Geometry check sheet. Reference: the model listing, model coordinates, mm. A direction names the side the tool comes from. Round coordinates to 2 decimals unless told otherwise and drop trailing zeros. Loops run counter-clockwise (first coordinate to the right, second up) from the corner with the lowest first, then second, coordinate; pieces in that order, holes last. Notation, with made-up numbers: (-6.5, -21) - (17.5, -21) arc R13 ccw to (17.5, 4) - close; hole circle Ø11 at (81.5, 87). An arc over 180 degrees is marked (long way). Write item = value, one per line.
Autodesk Inventor part; units mm, degrees
ref_plane "YZ Plane" through (0, 0, 0) normal (1, 0, 0) x (0, 1, 0)
ref_plane "XY Plane" through (0, 0, 0) normal (0, 0, 1) x (1, 0, 0)
sketch "Sketch1" plane through (0, 0, 0) normal (0, 0, 1) x (1, 0, 0)
  circle A0 centre (0, 0) radius 142.875
  circle A1 centre (0, 0) radius 149.225
  dimension "innerDiameter" = 285.75
  dimension "outerDiameter" = 298.45
extrude "Extrusion1" add sketch "Sketch1" along normal mid plane 19.05
sketch "Sketch2" plane through (0, 0, 0) normal (0, 0, 1) x (1, 0, 0)
  circle A0 centre (0, 0) radius 142.875 construction
  line L0 (0, 142.875) -> (0, 149.225) construction
  circle A1 centre (0, 0) radius 149.225 construction
  line L1 (0, 142.875) -> (44.45, 142.875)
  line L2 (44.45, 142.875) -> (44.45, 149.225)
  line L3 (44.45, 149.225) -> (19.05, 149.225)
  line L4 (0, 142.875) -> (-44.45, 142.875)
  line L5 (-44.45, 142.875) -> (-44.45, 149.225)
  line L6 (-44.45, 149.225) -> (19.05, 149.225)
  line L7 (371.6693, 35.081) -> (0, 0)
  dimension "halfBaseWidth" = 44.45
  dimension "baseThickness" = 6.35
  dimension "baseHeight" = 0
extrude "Extrusion2" add sketch "Sketch2" along normal mid plane 19.05
sketch "Sketch5" plane through (-44.45, 149.225, 9.525) normal (0, 1, 0) x (1, 0, 0)
  line L0 (0, 19.05) -> (0, 0)
  line L1 (88.9, 19.05) -> (88.9, 0)
  line L2 (0, 0) -> (88.9, 0)
  line L3 (88.9, 0) -> (88.9, 19.05)
  line L4 (88.9, 19.05) -> (0, 19.05)
  line L5 (0, 19.05) -> (0, 0)
  point P0 (44.45, 9.525)
  point P1 (0, 19.05)
extrude "Extrusion3" add sketch "Sketch5" along normal blind 63.5
sketch "Sketch7" plane through (0, 0, 9.525) normal (0, 0, 1) x (1, 0, 0)
  line L0 (-44.45, 142.875) -> (-44.45, 212.725)
  line L1 (-44.45, 212.725) -> (44.45, 212.725)
  line L2 (44.45, 142.875) -> (44.45, 212.725)
  line L3 (0, 212.725) -> (0, 149.1868) construction
  line L4 (-15.875, 197.104) -> (15.875, 197.104)
  line L5 (15.875, 197.104) -> (15.875, 206.375)
  line L6 (15.875, 206.375) -> (-15.875, 206.375)
  line L7 (-15.875, 206.375) -> (-15.875, 197.104)
  line L8 (-15.875, 197.104) -> (15.875, 206.375) construction
  line L9 (15.875, 197.104) -> (-15.875, 206.375) construction
  point P0 (0, 0)
  point P1 (-38.1, 144.2792)
  point P2 (38.1, 144.2792)
  point P3 (0, 201.7395)
  dimension "screwHoleWidth" = 31.75
  dimension "screwHoleHeight" = 9.271
  dimension "screwHoleSupportThickness" = 6.35
extrude "Extrusion4" cut sketch "Sketch7" against normal through all
sketch "Sketch6" plane through (-44.45, 212.725, 9.525) normal (0, 1, 0) x (1, 0, 0)
  point P0 (44.45, 9.525)
  point P1 (44.45, 9.525)
hole "Hole2" at (0, 212.725, 0) direction (0, -1, 0) diameter 6.7564 depth 6.35
ref_plane "Work Plane1" through (0, 0, 0) normal (-0.7071, 0.7071, 0) x (0, 0, 1)
ref_plane "Work Plane2" through (0, 0, 0) normal (0.7071, 0.7071, 0) x (0, 0, 1)
sketch "Sketch11" plane through (0, 0, 0) normal (0, 0, 1) x (1, 0, 0)
  arc A0 (-43.0678, 142.875) -> (43.0678, 142.875) centre (0, 0) ccw
  circle A1 centre (0, 0) radius 142.875
  line L0 (-214.9625, 214.9625) -> (217.3313, -217.3313)
  line L1 (-101.0279, 101.0279) -> (-96.5378, 105.518)
  line L2 (-101.0279, 101.0279) -> (-94.6779, 101.0279) construction
  line L3 (-96.5378, 105.518) -> (-114.4983, 123.4785)
  line L4 (-96.5378, 105.518) -> (-71.1378, 105.518) construction
  line L5 (-114.4983, 123.4785) -> (-118.9884, 118.9884)
  line L6 (-118.9884, 118.9884) -> (-101.0279, 101.0279)
  line L7 (-101.0279, 101.0279) -> (-105.518, 96.5378)
  line L8 (-105.518, 96.5378) -> (-123.4785, 114.4983)
  line L9 (-123.4785, 114.4983) -> (-118.9884, 118.9884)
  point P0 (38.1, 144.2792)
  point P1 (-38.1, 144.2792)
  point P2 (-109.9126, 100.9323)
  point P3 (-100.9323, 109.9126)
  dimension "d47" = 6.35
  dimension "d48" = 45
  dimension "d49" = 25.4
  dimension "d50" = 135
extrude "Extrusion7" add sketch "Sketch11" along normal mid plane 19.05 contours A0 L0 L5 L3 | A0 L8 L9 L0
sketch "Sketch12" plane through (-114.4983, 123.4785, -9.525) normal (0.7071, 0.7071, 0) x (-0.7071, 0.7071, 0)
  line L0 (0, 0) -> (0, 19.05)
  line L1 (-19.1852, 19.05) -> (0, 19.05)
  line L2 (-19.1852, 0) -> (-19.1852, 19.05)
  line L3 (0, 0) -> (-19.1852, 0)
  line L4 (-9.5926, 19.05) -> (-9.5926, 0) construction
  line L5 (0, 9.525) -> (-19.1852, 9.525) construction
  point P0 (-168.275, 9.525)
  point P1 (-9.5926, 9.525)
hole "Hole4" at (-107.7153, 116.6955, 0) direction (-0.7071, -0.7071, 0) diameter 5.1054 depth 12.7
pattern_circular "Circular Pattern1" count 4 over 360 about axis through (0, 0, -10) along (0, 0, 1) of "Extrusion7", "Hole4"
sketch "Sketch13" plane through (0, 0, 9.525) normal (0, 0, 1) x (1, 0, 0)
  line L0 (-15.875, 206.375) -> (15.875, 206.375)
  line L1 (-44.45, 212.725) -> (44.45, 212.725)
  line L2 (0, 208.915) -> (8.89, 208.915)
  line L3 (8.89, 208.915) -> (8.89, 206.375)
  line L4 (8.89, 206.375) -> (0, 206.375)
  line L5 (0, 208.915) -> (0, 206.375)
  line L6 (15.875, 206.375) -> (-15.875, 206.375)
  line L7 (0, 208.915) -> (-8.89, 208.915)
  line L8 (-8.89, 208.915) -> (-8.89, 206.375)
  point P0 (0, 0)
  dimension "d63" = 8.89
  dimension "d64" = 2.54
extrude "Extrusion8" cut sketch "Sketch13" against normal through all
sketch "Sketch14" plane through (0, 0, 9.525) normal (0, 0, 1) x (1, 0, 0)
  point P0 (0, 0)
sketch "Sketch15" plane through (0, 0, 0) normal (0, 0, 1) x (1, 0, 0)
  arc A0 (-43.0678, 142.875) -> (-100.9323, 109.9126) centre (0, 0) ccw
  line L0 (-43.0678, 142.875) -> (-44.45, 142.875)
  line L1 (44.45, 142.875) -> (43.0678, 142.875)
  arc A1 (100.9323, 109.9126) -> (43.0678, 142.875) centre (0, 0) ccw
  line L2 (-44.45, 142.875) -> (-44.45, 142.451)
  line L3 (-44.45, 142.875) -> (-43.0678, 142.875)
  line L4 (43.0678, 142.875) -> (44.45, 142.875)
  line L5 (44.45, 142.875) -> (44.45, 142.451)
  arc A2 (-43.0678, 142.875) -> (-44.45, 142.451) centre (0, 0) ccw
  arc A3 (44.45, 142.451) -> (43.0678, 142.875) centre (0, 0) ccw
extrude "Extrusion9" add sketch "Sketch15" along normal mid plane 19.05
sketch "Sketch16" plane through (0, 0, 0) normal (0, 0, 1) x (1, 0, 0)
  line L0 (44.45, 142.451) -> (44.45, 212.725)
  line L1 (-44.45, 142.451) -> (-44.45, 212.725)
  arc A0 (-44.45, 142.451) -> (-100.9323, 109.9126) centre (0, 0) ccw
  arc A1 (100.9323, 109.9126) -> (44.45, 142.451) centre (0, 0) ccw
  line L2 (0, 0) -> (-74.6125, 129.2326) construction
  line L3 (0, 0) -> (0, 149.225) construction
  line L4 (0, 0) -> (74.6125, 129.2326) construction
  line L5 (-44.45, 212.725) -> (-74.6125, 129.2326)
  line L6 (-44.45, 142.451) -> (-44.45, 212.725)
  line L7 (-44.45, 142.451) -> (-44.45, 212.725)
  line L8 (44.45, 212.725) -> (44.45, 142.451)
  line L9 (44.45, 212.725) -> (74.6125, 129.2326)
  arc A2 (74.6125, 129.2326) -> (44.45, 142.451) centre (0, 0) ccw
  arc A3 (-44.45, 142.451) -> (-74.6125, 129.2326) centre (0, 0) ccw
  dimension "d69" = 30
  dimension "d70" = 30
extrude "Extrusion10" add sketch "Sketch16" along normal mid plane 19.05
fillet "Fillet1" radius 3.175 2 edges at (-74.6125, 129.2326, 0) (74.6125, 129.2326, 0)
fillet "Fillet2" radius 3.175 2 edges at (-44.45, 212.725, 0) (44.45, 212.725, 0)
equation "\"outerDiameter\" = innerDiameter + 2 * ringThicknessRadius"
equation "\"d7\" = ringWidth"
equation "\"d51\" = ringWidth"
equation "\"d67\" = ringWidth"
equation "\"d71\" = ringWidth"
equation "\"ringThicknessRadius\" = 6.35"
properties part number "mount" material "PET Plastic"
(1) Set-up check for faces 5 (the flat face through (-109.13, -118.11, -2.25)), 6 (the flat face through (-118.11, 109.13, -2.25)), 7 (the flat face through (-4, 208.915, 0)): record each of +Z, -Z, +X, -X, +Y, -Y from which the full face is reachable in a straight line by a thin tool's end or side.
Answers follow:
face_5 = +Z, -Z, -Y
face_6 = +Z, -Z, -X
face_7 = +Z, -Z
(2) Mould release check, pull along X, two halves, no side actions. Record for faces 1 (the flat face through (-1, 212.725, -4)), 2 (the flat face through (-59.51, 171.04, -0.13)), 3 (the cylindrical face through (149.217, 1.552, -0.133)), 4 (the flat face through (-15.875, 202, 0)): pulls with the +X half, pulls with the -X half, needs draft (parallel to the pull), parting line crosses it, or undercut.
Answers follow:
face_1 = needs draft
face_2 = pulls with the -X half
face_3 = pulls with the +X half
face_4 = undercut
(3) Section check C-C (x = -25.5). Enter the section's corners in (y, z) (3 decimals), then the cut area to 3 significant figures.
Answers follow:
outline = (-147.03, -9.525) - (-140.581, -9.525) - (-140.581, 9.525) - (-147.03, 9.525) - close; (140.581, -9.525) - (212.725, -9.525) - (212.725, 9.525) - (140.581, 9.525) - close
area = 1,500 mm²
(4) Section check B-B (z = 6.5). State how many separate pieces and enclosed holes the cut face has, then the cut area to 3 significant figures.
Answers follow:
separate_pieces = 1
enclosed_holes = 2
area = 14,400 mm²
(5) Gauge pin test, flat ends, axial feed: pin 1 (3 mm diameter, centred on y = 207, z = -1, fed in from +X); pin 2 (4 mm diameter, centred on y = -23, z = -1.5, fed in from +X); pin 3 (6 mm diameter, centred on y = 59, z = 1.5, fed in from -X). Record the tip position at first contact, or that the pin passes through.
Answers follow:
pin_1 = 47.06
pin_2 = 147.74
pin_3 = -138.32
(6) Section check A-A (y = 0). Enter the section's corners in (x, z) (3 decimals).
Answers follow:
outline = (-149.225, -9.525) - (-142.875, -9.525) - (-142.875, 9.525) - (-149.225, 9.525) - close; (142.875, -9.525) - (149.225, -9.525) - (149.225, 9.525) - (142.875, 9.525) - close
(7) Scan lines: L1, parallel to X at y = 2.5, z = 5.5; L2, parallel to Y at x = 0, z = -2 (3 decimals); L3, parallel to Z at x = 0, y = 211.65 (3 decimals). Record each from-to range of solid material in increasing order. Write a range as [from, to].
Answers follow:
L1 = [-149.2, -142.85], [142.85, 149.2]
L2 = [-149.225, -142.875], [142.875, 197.104]
L3 = [-9.525, -3.378], [3.378, 9.525]
